```python
from build123d import *

# Parameters (mm, degrees)
SKETCH_1_W                   = 432
SKETCH_1_H                   = 330
EXTRUDE_1_DEPTH              = 4
HOLE_WIZARD_M4_1_AT_2_COUNT  = 2
HOLE_WIZARD_M4_1_AT_2_PITCH  = 90
HOLE_WIZARD_M4_1_AT_3_COUNT  = 2
HOLE_WIZARD_M4_1_AT_3_PITCH  = 180
HOLE_WIZARD_M4_1_AT_4_COUNT  = 2
HOLE_WIZARD_M4_1_AT_4_PITCH  = 270
HOLE_WIZARD_M4_1_AT_5_COUNT  = 2
HOLE_WIZARD_M4_1_AT_5_PITCH  = 293.48296373
HOLE_WIZARD_M4_1_AT_6_COUNT  = 2
HOLE_WIZARD_M4_1_AT_6_PITCH  = 327.811302429
HOLE_WIZARD_M4_1_AT_7_COUNT  = 2
HOLE_WIZARD_M4_1_AT_7_PITCH  = 399.424899074
HOLE_WIZARD_M4_1_AT_8_COUNT  = 2
HOLE_WIZARD_M4_1_AT_8_PITCH  = 492.31316253
HOLE_WIZARD_M4_1_AT_9_COUNT  = 2
HOLE_WIZARD_M4_1_AT_9_PITCH  = 499.299509313
HOLE_WIZARD_M4_1_AT_10_COUNT = 2
HOLE_WIZARD_M4_1_AT_10_PITCH = 456.946386352
HOLE_WIZARD_M4_1_AT_11_COUNT = 2
HOLE_WIZARD_M4_1_AT_11_PITCH = 429.534631898
HOLE_WIZARD_M4_1_AT_12_COUNT = 2
HOLE_WIZARD_M4_1_AT_12_PITCH = 420
HOLE_WIZARD_M4_1_AT_13_COUNT = 2
HOLE_WIZARD_M4_1_AT_13_PITCH = 396.726606116
HOLE_WIZARD_M4_1_AT_14_COUNT = 2
HOLE_WIZARD_M4_1_AT_14_PITCH = 273.056770654
HOLE_WIZARD_M4_1_AT_15_COUNT = 2
HOLE_WIZARD_M4_1_AT_15_PITCH = 149.933318512
HOLE_WIZARD_M4_1_AT_16_COUNT = 2
HOLE_WIZARD_M4_1_AT_16_PITCH = 33.941125497
FILLET_1_R                   = 2


with BuildPart() as part:
    # 草圖1 → 填料-伸長1 (new body)
    with BuildSketch(Plane(origin=(0, 0, 0), x_dir=(1, 0, 0), z_dir=(0, 1, 0))):
        with Locations((216, 165)):
            Rectangle(SKETCH_1_W, SKETCH_1_H)
    extrude(amount=EXTRUDE_1_DEPTH)

    # 草圖2 → M4 六角凹錐坑螺釘的錐孔1 (revolve, cut)
    with BuildSketch(Plane(origin=(6, 4, -300), x_dir=(0, 0, 1), z_dir=(1, 0, 0))):
        Polygon((0, 0), (0, 4), (2.25, 4), (2.25, 2.23), (4.48, 0), align=None)
    hole_wizard_m4_1 = revolve(axis=Axis((6, 10.35, -300), (0, -1, 0)), mode=Mode.SUBTRACT)

    # M4 六角凹錐坑螺釘的錐孔1 at 2: M4 六角凹錐坑螺釘的錐孔1 ×2
    with Locations(*[(0, 0, i * HOLE_WIZARD_M4_1_AT_2_PITCH) for i in range(1, HOLE_WIZARD_M4_1_AT_2_COUNT)]):
        add(hole_wizard_m4_1, mode=Mode.SUBTRACT)

    # M4 六角凹錐坑螺釘的錐孔1 at 3: M4 六角凹錐坑螺釘的錐孔1 ×2
    with Locations(*[(0, 0, i * HOLE_WIZARD_M4_1_AT_3_PITCH) for i in range(1, HOLE_WIZARD_M4_1_AT_3_COUNT)]):
        add(hole_wizard_m4_1, mode=Mode.SUBTRACT)

    # M4 六角凹錐坑螺釘的錐孔1 at 4: M4 六角凹錐坑螺釘的錐孔1 ×2
    with Locations(*[(0, 0, i * HOLE_WIZARD_M4_1_AT_4_PITCH) for i in range(1, HOLE_WIZARD_M4_1_AT_4_COUNT)]):
        add(hole_wizard_m4_1, mode=Mode.SUBTRACT)

    # M4 六角凹錐坑螺釘的錐孔1 at 5: M4 六角凹錐坑螺釘的錐孔1 ×2
    with Locations(*[Vector(0.081776467, 0, 0.996650696) * (i * HOLE_WIZARD_M4_1_AT_5_PITCH) for i in range(1, HOLE_WIZARD_M4_1_AT_5_COUNT)]):
        add(hole_wizard_m4_1, mode=Mode.SUBTRACT)

    # M4 六角凹錐坑螺釘的錐孔1 at 6: M4 六角凹錐坑螺釘的錐孔1 ×2
    with Locations(*[Vector(0.451479247, 0, 0.89228162) * (i * HOLE_WIZARD_M4_1_AT_6_PITCH) for i in range(1, HOLE_WIZARD_M4_1_AT_6_COUNT)]):
        add(hole_wizard_m4_1, mode=Mode.SUBTRACT)

    # M4 六角凹錐坑螺釘的錐孔1 at 7: M4 六角凹錐坑螺釘的錐孔1 ×2
    with Locations(*[Vector(0.680979079, 0, 0.73230287) * (i * HOLE_WIZARD_M4_1_AT_7_PITCH) for i in range(1, HOLE_WIZARD_M4_1_AT_7_COUNT)]):
        add(hole_wizard_m4_1, mode=Mode.SUBTRACT)

    # M4 六角凹錐坑螺釘的錐孔1 at 8: M4 六角凹錐坑螺釘的錐孔1 ×2
    with Locations(*[Vector(0.804366062, 0, 0.594134023) * (i * HOLE_WIZARD_M4_1_AT_8_PITCH) for i in range(1, HOLE_WIZARD_M4_1_AT_8_COUNT)]):
        add(hole_wizard_m4_1, mode=Mode.SUBTRACT)

    # M4 六角凹錐坑螺釘的錐孔1 at 9: M4 六角凹錐坑螺釘的錐孔1 ×2
    with Locations(*[Vector(0.841178475, 0, 0.540757591) * (i * HOLE_WIZARD_M4_1_AT_9_PITCH) for i in range(1, HOLE_WIZARD_M4_1_AT_9_COUNT)]):
        add(hole_wizard_m4_1, mode=Mode.SUBTRACT)

    # M4 六角凹錐坑螺釘的錐孔1 at 10: M4 六角凹錐坑螺釘的錐孔1 ×2
    with Locations(*[Vector(0.91914503, 0, 0.393919299) * (i * HOLE_WIZARD_M4_1_AT_10_PITCH) for i in range(1, HOLE_WIZARD_M4_1_AT_10_COUNT)]):
        add(hole_wizard_m4_1, mode=Mode.SUBTRACT)

    # M4 六角凹錐坑螺釘的錐孔1 at 11: M4 六角凹錐坑螺釘的錐孔1 ×2
    with Locations(*[Vector(0.977802414, 0, 0.209529089) * (i * HOLE_WIZARD_M4_1_AT_11_PITCH) for i in range(1, HOLE_WIZARD_M4_1_AT_11_COUNT)]):
        add(hole_wizard_m4_1, mode=Mode.SUBTRACT)

    # M4 六角凹錐坑螺釘的錐孔1 at 12: M4 六角凹錐坑螺釘的錐孔1 ×2
    with Locations(*[(i * HOLE_WIZARD_M4_1_AT_12_PITCH, 0, 0) for i in range(1, HOLE_WIZARD_M4_1_AT_12_COUNT)]):
        add(hole_wizard_m4_1, mode=Mode.SUBTRACT)

    # M4 六角凹錐坑螺釘的錐孔1 at 13: M4 六角凹錐坑螺釘的錐孔1 ×2
    with Locations(*[Vector(0.998168497, 0, -0.06049506) * (i * HOLE_WIZARD_M4_1_AT_13_PITCH) for i in range(1, HOLE_WIZARD_M4_1_AT_13_COUNT)]):
        add(hole_wizard_m4_1, mode=Mode.SUBTRACT)

    # M4 六角凹錐坑螺釘的錐孔1 at 14: M4 六角凹錐坑螺釘的錐孔1 ×2
    with Locations(*[Vector(0.99612985, 0, -0.08789381) * (i * HOLE_WIZARD_M4_1_AT_14_PITCH) for i in range(1, HOLE_WIZARD_M4_1_AT_14_COUNT)]):
        add(hole_wizard_m4_1, mode=Mode.SUBTRACT)

    # M4 六角凹錐坑螺釘的錐孔1 at 15: M4 六角凹錐坑螺釘的錐孔1 ×2
    with Locations(*[Vector(0.987105478, 0, -0.160071159) * (i * HOLE_WIZARD_M4_1_AT_15_PITCH) for i in range(1, HOLE_WIZARD_M4_1_AT_15_COUNT)]):
        add(hole_wizard_m4_1, mode=Mode.SUBTRACT)

    # M4 六角凹錐坑螺釘的錐孔1 at 16: M4 六角凹錐坑螺釘的錐孔1 ×2
    with Locations(*[Vector(0.707106781, 0, -0.707106781) * (i * HOLE_WIZARD_M4_1_AT_16_PITCH) for i in range(1, HOLE_WIZARD_M4_1_AT_16_COUNT)]):
        add(hole_wizard_m4_1, mode=Mode.SUBTRACT)

    # 圓角1
    fillet_1_edges = [part.edges().sort_by_distance(p)[0] for p in [
        (216, 4, 0),
    ]]
    fillet(fillet_1_edges, radius=FILLET_1_R)


solid = part.part
```
Check sheet for the modelled part. Datum: model origin and axes. Units: mm. Coordinates: 2 decimals unless noted, no trailing zeros. Write item = value, one per line. Start each with the question number.
1) Material ranges on L1, parallel to Z at x = 6, y = 0.5; L2, parallel to X at y = 1.25, z = -210; L3, parallel to X at y = 0.7, z = -7.5, recorded low to high.
2) Go/stop test with flat-tipped pins: P1, Ø5, axis at x = 6, z = -120, coming from the +Y side; P2, Ø5, axis at x = 426, z = -300, coming from the -Y side. Record where each tip stops, or that it passes through.
3) Mould release check, pull along Z, two halves, no side actions. Record for faces 1 (the flat face through (213, 0, -167)), 2 (the conical face through (275.63, 1.91, -324.31)): +Z half, -Z half, draft (parallel to the pull), parting line (faces both ways), or undercut.
Ans:
q1.L1 = -330 to -302.25, -297.75 to -212.25, -207.75 to -122.25, -117.75 to -32.25, -27.75 to 0
q1.L2 = 0 to 3.75, 8.25 to 423.75, 428.25 to 432
q1.L3 = 0 to 27.75, 32.25 to 151.75, 156.25 to 275.75, 280.25 to 399.75, 404.25 to 432
q2.P1 = 2.02
q2.P2 = 0
q3.face_1 = draft
q3.face_2 = undercut
